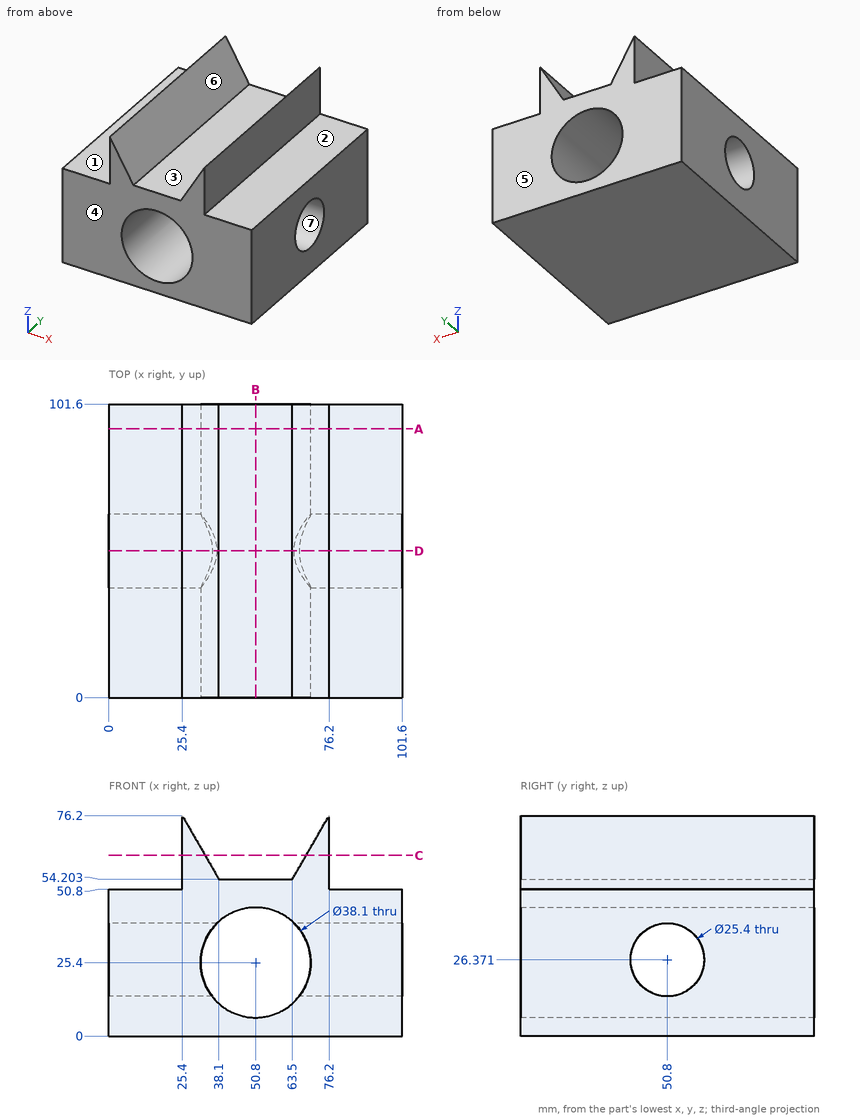
Here's the drawing with two shaded views (mm, measured from the low corner). I have some questions. A direction names the side the tool comes from. Round coordinates to 2 decimals unless told otherwise and drop trailing zeros. Order: outer loops, then holes, each group sorted by start corner. A loop starts at its lowest first (then second) coordinate and runs counter-clockwise, first axis right, second up. Notation, with made-up numbers: M 74.25,42 L 82.25,42 A17 cw 82.25,47 Z; hole C 29.5,-26.75 d8. An arc over 180 degrees is marked long. Answer in a Markdown table with one row per item.
Item 1: I'm going to push flat-ended pins straight in: pin 1 (7.5 mm diameter, centred on y = 31.5, z = 61.5, fed in from +X); pin 2 (7.5 mm diameter, centred on y = 57, z = 62.5, fed in from -X); pin 3 (20.5 mm diameter, centred on x = 57, y = 68, fed in from +Z); pin 4 (8 mm diameter, centred on x = 66, z = 61.5, fed in from -Y). Where does each tip first touch, or does it pass through?
A:
| item | result |
|---|---|
| pin 1 | stops at x = 76.2 |
| pin 2 | stops at x = 25.4 |
| pin 3 | stops at z = 60.7 |
| pin 4 | stops at y = 0 |
Item 2: Thinking about a two-plate mould opening in Y: for the marked faces 4, 5, 6 and 7, which applies, +Y half, -Y half, draft (parallel to the pull), parting line (faces both ways), or undercut?
A:
| item | result |
|---|---|
| face 4 | -Y half |
| face 5 | +Y half |
| face 6 | draft |
| face 7 | undercut |
Item 3: Imagine slicing it at D-D, the plane y = 50.8. Write out the boundary of the cut face in (x, z).
A:
| item | result |
|---|---|
| outline | M 0,0 L 101.6,0 L 101.6,13.67 L 65.81,13.67 A19.05 cw 35.79,13.67 L 0,13.67 Z; M 0,39.07 L 37.53,39.07 A19.05 cw 64.07,39.07 L 101.6,39.07 L 101.6,50.8 L 76.2,50.8 L 76.2,76.2 L 63.5,54.2 L 38.1,54.2 L 25.4,76.2 L 25.4,50.8 L 0,50.8 Z |
Item 4: Imagine slicing it at C-C, the plane z = 62.5. Write out the boundary of the cut face in (x, y).
A:
| item | result |
|---|---|
| outline | M 25.4,0 L 33.31,0 L 33.31,101.6 L 25.4,101.6 Z; M 68.29,0 L 76.2,0 L 76.2,101.6 L 68.29,101.6 Z |
Item 5: If I drill on L1, parallel to Z at x = 50.8, y = 57; L2, parallel to Y at x = 21, z = 27 (1 decimal); L3, parallel to Z at x = 91.5, y = 50.8, over which ranges is the centre line in solid material (lowest first)? Write a range as from..to.
A:
| item | result |
|---|---|
| L1 | z = 0..6.35, 44.45..54.2 |
| L2 | y = 0..38.1, 63.5..101.6 |
| L3 | z = 0..13.67, 39.07..50.8 |
Item 6: Imagine slicing it at A-A, the plane y = 93. Write out the boundary of the cut face in (x, z), and give its area (3 significant figures).
A:
| item | result |
|---|---|
| outline | M 0,0 L 101.6,0 L 101.6,50.8 L 76.2,50.8 L 76.2,76.2 L 63.5,54.2 L 38.1,54.2 L 25.4,76.2 L 25.4,50.8 L 0,50.8 Z; hole C 50.8,25.4 d38.1 |
| area | 4,470 mm2 |
Item 7: For the marked faces 1, 2 and 3, which set-ups out of +Z, -Z, +X, -X, +Y, -Y let a thin tool reach every point of the face, with its end or its side?
A:
| item | result |
|---|---|
| face 1 | +Z, -X, +Y, -Y |
| face 2 | +Z, +X, +Y, -Y |
| face 3 | +Z, +Y, -Y |
Item 8: Imagine slicing it at B-B, the plane x = 50.8. Write out the boundary of the cut face in (y, z).
A:
| item | result |
|---|---|
| outline | M 0,0 L 101.6,0 L 101.6,6.35 L 0,6.35 Z; M 0,44.45 L 101.6,44.45 L 101.6,54.2 L 0,54.2 Z |
